Geometry check sheet. Reference: the model listing, model coordinates, mm. Face numbers are marked on the shaded views. Round coordinates to 2 decimals unless told otherwise and drop trailing zeros. Order: outer loops, then holes, each group sorted by start corner. A loop starts at its lowest first (then second) coordinate and runs counter-clockwise, first axis right, second up. Notation, with made-up numbers: (-5.75, 85) - (48.25, 85) arc R14 cw to (48.25, 95) - close; hole circle Ø4 at (89, 62). An arc over 180 degrees is marked (long way). Return JSON: item names as keys, results as strings. Group by question number.
Q1. Sectioned sample at D-D, the plane y = 7.5. Record the cut outline in (x, z), then the cut area to 3 significant figures.
Q2. Sectioned sample at A-A, the plane y = 20. Record the cut outline in (x, z).
Q3. Sectioned sample at C-C, the plane x = 0. Record the cut outline in (y, z), then the cut area to 3 significant figures.
Q4. Draft check along X on the marked faces 1, 2 and 3. Enter one of: pulls with the +X half, pulls with the -X half, needs draft (parallel to the pull), parting line crosses it, or undercut.
Q5. Gauge pin test, flat ends, axial feed: pin 1 Ø10 at (x, y) = (-17.5, -2.5) entering from +Z; pin 2 Ø1.5 at (x, y) = (8.5, -12) entering from -Z. Record the tip position at first contact, or that the pin passes through.
Q6. Sectioned sample at B-B, the plane z = 1.5. Give the number of separate pieces and of enclosed holes in the cut face, then the cut area to 3 significant figures.
Q7. Material ranges on line 1 along Y through (x, z) = (0, 2.4); line 2 along Y through (x, z) = (14, 0.8); line 3 along X through (y, z) = (-10, 1.05), recorded low to high.
```python
from build123d import *

# Parameters (mm, degrees)
F0_R     = 25
F1_DEPTH = 3
F2_R     = 2.25
F3_DEPTH = 25
F4_R     = 10
F5_DEPTH = 25


with BuildPart() as f1:
    # F0 (on Top) → F1 (new body)
    with BuildSketch(Plane.XY):
        Circle(F0_R)
    extrude(amount=F1_DEPTH)

    # F2 (on face) → F3 (cut)
    with BuildSketch(Plane.XY.offset(3)):
        with Locations((0, 15)):
            Circle(F2_R)
        with Locations((-12.990381, 7.5)):
            Circle(F2_R)
        with Locations((-12.990381, -7.5)):
            Circle(F2_R)
        with Locations((0, -15)):
            Circle(F2_R)
        with Locations((12.990381, -7.5)):
            Circle(F2_R)
        with Locations((12.990381, 7.5)):
            Circle(F2_R)
    extrude(amount=-F3_DEPTH, mode=Mode.SUBTRACT)

    # F4 (on face) → F5 (cut)
    with BuildSketch(Plane.XY.offset(3)):
        with Locations((0, 20)):
            Circle(F4_R)
        with Locations((-17.320508, -10)):
            Circle(F4_R)
        with Locations((17.320508, -10)):
            Circle(F4_R)
    extrude(amount=-F5_DEPTH, mode=Mode.SUBTRACT)


solid = f1.part
```
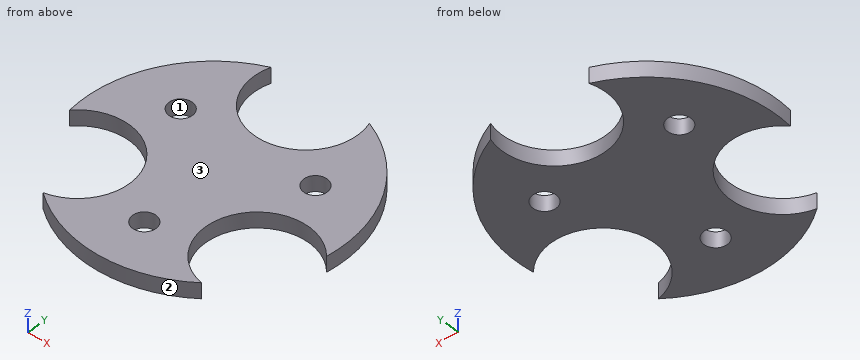
Reply:
{
 "1": {"outline": "(-23.85, 0) - (-15.24, 0) - (-15.24, 3) - (-23.85, 3) - close; (-10.74, 0) - (10.74, 0) - (10.74, 3) - (-10.74, 3) - close; (15.24, 0) - (23.85, 0) - (23.85, 3) - (15.24, 3) - close", "area": "116 mm^2"},
 "2": {"outline": "(-15, 0) - (-10, 0) - (-10, 3) - (-15, 3) - close; (10, 0) - (15, 0) - (15, 3) - (10, 3) - close"},
 "3": {"outline": "(-25, 0) - (-17.25, 0) - (-17.25, 3) - (-25, 3) - close; (-12.75, 0) - (10, 0) - (10, 3) - (-12.75, 3) - close", "area": "91.5 mm^2"},
 "4": {"face 1": "undercut", "face 2": "parting line crosses it", "face 3": "needs draft"},
 "5": {"pin 1": "z = 3", "pin 2": "through"},
 "6": {"separate pieces": "1", "enclosed holes": "3", "area": "1,190 mm^2"},
 "7": {"line 1": "-25 to -17.25, -12.75 to 10", "line 2": "-20.71 to -19.43, -0.57 to 5.49, 9.51 to 20.71", "line 3": "-7.32 to 7.32"}
}
